For this review, take the finished solid that the model builds, in its own axes (mm). A direction names the side the tool comes from. Coordinates: 2 decimals unless noted, no trailing zeros. Loops run counter-clockwise (first coordinate to the right, second up) from the corner with the lowest first, then second, coordinate; pieces in that order, holes last.
```python
from build123d import *

# Parameters (mm, degrees)
SKETCH1_R               = 2.159
SKETCH1_R_2             = 28.5115
BOSS_EXTRUDE1_DEPTH     = 9.7155
SKETCH1_3_R             = 28.5115
SKETCH1_3_R_2           = 23.8125
EXTENDED_BEZEL_DEPTH    = 13.0175
SKETCH1_5_R             = 28.5115
SKETCH1_5_R_2           = 23.8125
BOSS_EXTRUDE4_DEPTH     = 6.35
SKETCH2_R               = 25.3365
CUT_EXTRUDE1_DEPTH      = 7.35
CUT_EXTRUDE1_DEPTH_BACK = 9.7155
FILLET1_R               = 1.1938
SKETCH3_R               = 28.5115
CUT_EXTRUDE2_DEPTH      = 7.35


with BuildPart() as part:
    # Sketch1 → Boss-Extrude1 (new body)
    with BuildSketch(Plane.XY):
        with BuildLine():
            ThreePointArc((-24.49722379, -28.024879905), (-26.788104009, -26.788104009), (-28.024879905, -24.49722379))
            Line((-28.024879905, -24.49722379), (-30.1625, -14.199031657))
            Line((-30.1625, -14.199031657), (-30.1625, 14.199031657))
            Line((-30.1625, 14.199031657), (-28.024879905, 24.49722379))
            ThreePointArc((-28.024879905, 24.49722379), (-26.788104009, 26.788104009), (-24.49722379, 28.024879905))
            Line((-24.49722379, 28.024879905), (-14.199031657, 30.1625))
            Line((-14.199031657, 30.1625), (14.199031657, 30.1625))
            Line((14.199031657, 30.1625), (24.441349319, 28.268787691))
            ThreePointArc((24.441349319, 28.268787691), (26.949748619, 26.949748619), (28.268787691, 24.441349319))
            Line((28.268787691, 24.441349319), (30.1625, 14.199031657))
            Line((30.1625, 14.199031657), (30.1625, -14.199031657))
            Line((30.1625, -14.199031657), (28.024879905, -24.49722379))
            ThreePointArc((28.024879905, -24.49722379), (26.788104009, -26.788104009), (24.49722379, -28.024879905))
            Line((24.49722379, -28.024879905), (14.199031657, -30.1625))
            Line((14.199031657, -30.1625), (-14.199031657, -30.1625))
            Line((-14.199031657, -30.1625), (-24.49722379, -28.024879905))
        make_face()
        with Locations((-23.573172318, -23.573172318)):
            Circle(SKETCH1_R, mode=Mode.SUBTRACT)
        with Locations((23.573172318, -23.573172318)):
            Circle(SKETCH1_R, mode=Mode.SUBTRACT)
        with Locations((23.573172318, 23.573172318)):
            Circle(SKETCH1_R, mode=Mode.SUBTRACT)
        with Locations((-23.573172318, 23.573172318)):
            Circle(SKETCH1_R, mode=Mode.SUBTRACT)
        Circle(SKETCH1_R_2, mode=Mode.SUBTRACT)
        with BuildLine():
            Line((28.268787691, 24.441349319), (30.1625, 14.199031657))
            Line((30.1625, 14.199031657), (30.1625, 25.3873))
            ThreePointArc((30.1625, 25.3873), (28.763876302, 28.763876302), (25.3873, 30.1625))
            Line((25.3873, 30.1625), (14.199031657, 30.1625))
            Line((14.199031657, 30.1625), (24.441349319, 28.268787691))
            ThreePointArc((24.441349319, 28.268787691), (26.949748619, 26.949748619), (28.268787691, 24.441349319))
        make_face()
        with BuildLine():
            Line((-30.1625, 25.3873), (-30.1625, 14.199031657))
            Line((-30.1625, 14.199031657), (-28.024879905, 24.49722379))
            ThreePointArc((-28.024879905, 24.49722379), (-26.788104009, 26.788104009), (-24.49722379, 28.024879905))
            Line((-24.49722379, 28.024879905), (-14.199031657, 30.1625))
            Line((-14.199031657, 30.1625), (-25.3873, 30.1625))
            ThreePointArc((-25.3873, 30.1625), (-28.763876302, 28.763876302), (-30.1625, 25.3873))
        make_face()
        with BuildLine():
            Line((-25.3873, -30.1625), (-14.199031657, -30.1625))
            Line((-14.199031657, -30.1625), (-24.49722379, -28.024879905))
            ThreePointArc((-24.49722379, -28.024879905), (-26.788104009, -26.788104009), (-28.024879905, -24.49722379))
            Line((-28.024879905, -24.49722379), (-30.1625, -14.199031657))
            Line((-30.1625, -14.199031657), (-30.1625, -25.3873))
            ThreePointArc((-30.1625, -25.3873), (-28.763876302, -28.763876302), (-25.3873, -30.1625))
        make_face()
        with BuildLine():
            Line((24.49722379, -28.024879905), (14.199031657, -30.1625))
            Line((14.199031657, -30.1625), (25.3873, -30.1625))
            ThreePointArc((25.3873, -30.1625), (28.763876302, -28.763876302), (30.1625, -25.3873))
            Line((30.1625, -25.3873), (30.1625, -14.199031657))
            Line((30.1625, -14.199031657), (28.024879905, -24.49722379))
            ThreePointArc((28.024879905, -24.49722379), (26.788104009, -26.788104009), (24.49722379, -28.024879905))
        make_face()
    extrude(amount=BOSS_EXTRUDE1_DEPTH)

    # Sketch1_3 → Extended Bezel (add)
    with BuildSketch(Plane.XY):
        Circle(SKETCH1_3_R)
        Circle(SKETCH1_3_R_2, mode=Mode.SUBTRACT)
    extrude(amount=EXTENDED_BEZEL_DEPTH)

    # Sketch1_5 → Boss-Extrude4 (add)
    with BuildSketch(Plane.XY):
        Circle(SKETCH1_5_R)
        Circle(SKETCH1_5_R_2, mode=Mode.SUBTRACT)
    extrude(amount=-BOSS_EXTRUDE4_DEPTH)

    # Sketch2 → Cut-Extrude1 (cut, two sides)
    with BuildSketch(Plane(origin=(0, 0, 0), x_dir=(-1, 0, 0), z_dir=(0, 0, -1))) as cut_extrude1_sk:
        Circle(SKETCH2_R)
    extrude(amount=CUT_EXTRUDE1_DEPTH, mode=Mode.SUBTRACT)
    extrude(cut_extrude1_sk.sketch, amount=-CUT_EXTRUDE1_DEPTH_BACK, mode=Mode.SUBTRACT)

    # Fillet1
    fillet1_edges = [part.edges().sort_by_distance(p)[0] for p in [
        (28.763876302, -28.763876302, 9.7155),
        (30.1625, 0, 9.7155),
        (28.763876302, 28.763876302, 9.7155),
        (0, 30.1625, 9.7155),
        (-28.763876302, 28.763876302, 9.7155),
        (-30.1625, 0, 9.7155),
        (-23.8125, 0, 13.0175),
        (-28.5115, 0, 13.0175),
        (-28.763876302, -28.763876302, 9.7155),
        (0, -30.1625, 9.7155),
    ]]
    fillet(fillet1_edges, radius=FILLET1_R)

    # Sketch3 → Cut-Extrude2 (cut, through all)
    with BuildSketch(Plane(origin=(0, 0, 0), x_dir=(-1, 0, 0), z_dir=(0, 0, -1))):
        Circle(SKETCH3_R)
    extrude(amount=CUT_EXTRUDE2_DEPTH, mode=Mode.SUBTRACT)


solid = part.part
```
Q1. Consider section A-A (x = 0). State the section outline as (y, z) points, then the cut area to 3 significant figures.
Q2. Machinability: for faces 1 (the face through (-23.854, 25.714, 4.79)), 2 (the face through (-13.621, 21.364, 4.926)), 3 (the face through (28, -6.3, 9.716)), which of the approach directions +Z, -Z, +X, -X, +Y, -Y give a long, thin tool a straight path to every point of the face, cutting with its end or side? Answer none if there is none.
Q3. Wall thickness on probe 1 along Y at (x, z) = (25.5, 4.25); probe 2 along Y at (x, z) = (0, 7.75); probe 3 along Z at (x, y) = (-25, -21): over which ranges is each line inside the solid? List them lowest first.
Q4. For pin 1 Ø4 at (x, y) = (23.57, -23.57) entering from -Z; pin 2 Ø4 at (x, y) = (-6, 21.5) entering from -Z; pin 3 Ø5.5 at (x, y) = (-23.57, -23.57) entering from +Z; pin 4 Ø1 at (y, z) = (-15, 9.5) entering from -X, all flat-tipped, find the tip position at first contact; note any pin that passes through.
Q5. Consider section C-C (z = 7). State the section outline as (x, y) points, then the cut area to 3 significant figures.
Model answer:
1. outline: (-30.16, 0) - (-25.34, 0) - (-25.34, 9.72) - (-23.81, 9.72) - (-23.81, 11.82) arc R1.19 ccw to (-25.01, 13.02) - (-27.32, 13.02) arc R1.19 ccw to (-28.51, 11.82) - (-28.51, 9.72) - (-28.97, 9.72) arc R1.19 ccw to (-30.16, 8.52) - close; (23.81, 9.72) - (25.34, 9.72) - (25.34, 0) - (30.16, 0) - (30.16, 8.52) arc R1.19 ccw to (28.97, 9.72) - (28.51, 9.72) - (28.51, 11.82) arc R1.19 ccw to (27.32, 13.02) - (25.01, 13.02) arc R1.19 ccw to (23.81, 11.82) - close
1. area: 123 mm2
2. face 1: +Z, -Z
2. face 2: -Z
2. face 3: +Z
3. probe 1: y = -30.16 to -24.55, -22.6 to 22.6, 24.55 to 30.16
3. probe 2: y = -30.16 to -25.34, 25.34 to 30.16
3. probe 3: z = 0 to 9.72
4. pin 1: passes through
4. pin 2: stops at z = 9.72
4. pin 3: stops at z = 9.72
4. pin 4: stops at x = -30.06
5. outline: (-30.16, -25.39) arc R4.78 ccw to (-25.39, -30.16) - (25.39, -30.16) arc R4.78 ccw to (30.16, -25.39) - (30.16, 25.39) arc R4.78 ccw to (25.39, 30.16) - (-25.39, 30.16) arc R4.78 ccw to (-30.16, 25.39) - close; hole circle Ø4.32 at (-23.57, -23.57); hole circle Ø4.32 at (-23.57, 23.57); hole circle Ø50.67 at (0, 0); hole circle Ø4.32 at (23.57, -23.57); hole circle Ø4.32 at (23.57, 23.57)
5. area: 1,540 mm2
